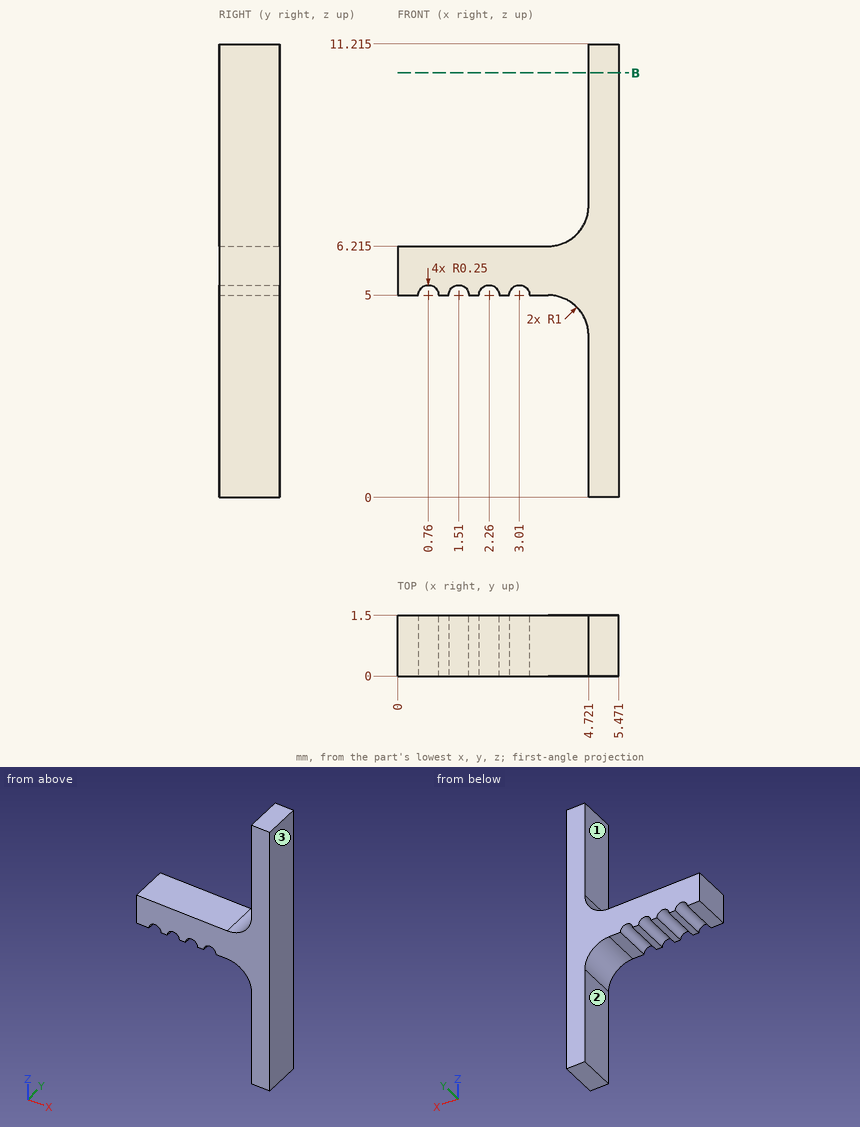
Geometry: see drawing. Coordinates: mm, zero at the bounding-box minimum. A direction names the side the tool comes from. Round coordinates to 2 decimals unless told otherwise and drop trailing zeros. Order: outer loops, then holes, each group sorted by start corner. A loop starts at its lowest first (then second) coordinate and runs counter-clockwise, first axis right, second up. Notation, with made-up numbers: (-23, -34) - (10, -34) arc R8 ccw to (10, -25) - close; hole circle Ø3 at (52.25, 38). An arc over 180 degrees is marked (long way). Use a Markdown table: item, result. Add a question column.
1. Section query B-B (z = 10.5). Return the cut outline in (x, y).
2. Set-up query: the marked faces 1, 2 and 3. Return all of +Z, -Z, +X, -X, +Y, -Y with unobstructed straight access to the full face (end or side cutting, diameter ignored); none if empty.
3. Line query: probe 1 along X at (y, z) = (1.05, 1.25); probe 2 along Z at (x, y) = (0.25, 0.55) (1 decimal); probe 3 along Z at (x, y) = (2.3, 0.25) (1 decimal). Output: solid intervals per line, ascending.
4. First-contact query: pin 1 (0.8 mm diameter, centred on x = 2, y = 0.5, fed in from +Z) (3 decimals); pin 2 (0.8 mm diameter, centred on y = 0.5, z = 9.5, fed in from -X). Flat tips, straight axial feed; report the tip coordinate or a pass-through.
Derived:
| question | item | result |
|---|---|---|
| 1 | outline | (4.72, 0) - (5.47, 0) - (5.47, 1.5) - (4.72, 1.5) - close |
| 2 | face 1 | +Z, -X, +Y, -Y |
| 2 | face 2 | -Z, -X, +Y, -Y |
| 2 | face 3 | +Z, -Z, +X, +Y, -Y |
| 3 | probe 1 | 4.72 to 5.47 |
| 3 | probe 2 | 5 to 6.2 |
| 3 | probe 3 | 5.2 to 6.2 |
| 4 | pin 1 | z = 6.215 |
| 4 | pin 2 | x = 4.72 |
